Design review of the part built by this model. Coordinates are the model's own, in mm. A direction names the side the tool comes from. Round coordinates to 2 decimals unless told otherwise and drop trailing zeros. Loops run counter-clockwise (first coordinate to the right, second up) from the corner with the lowest first, then second, coordinate; pieces in that order, holes last. Notation, with made-up numbers: (37, 14.25) -> (91, 14.25) arc R7 ccw to (91, 20.25) -> close; hole circle Ø2 at (-39.75, 18). An arc over 180 degrees is marked (long way). Use a Markdown table: item, result. Add a question column.
from build123d import *

# Parameters (mm, degrees)
SALIENTE_EXTRUIR1_DEPTH = 4
CORTAR_EXTRUIR4_DEPTH   = 5
CROQUIS10_R             = 1.5
CORTAR_EXTRUIR5_DEPTH   = 5
CROQUIS12_R             = 2.575
CORTAR_EXTRUIR6_DEPTH   = 5


with BuildPart() as part:
    # Croquis1 → Saliente-Extruir1 (new body)
    with BuildSketch(Plane(origin=(0, 0, 0), x_dir=(1, 0, 0), z_dir=(0, 1, 0))):
        with BuildLine():
            Line((-18.025, -25), (18.025, -25))
            ThreePointArc((18.025, -25), (21.560533906, -23.535533906), (23.025, -20))
            Line((23.025, -20), (23.025, -14))
            Line((23.025, -14), (29.025, -14))
            Line((29.025, -14), (29.025, -8))
            Line((29.025, -8), (23.025, -8))
            Line((23.025, -8), (23.025, -1.55))
            Line((23.025, -1.55), (20.975, -1.55))
            Line((20.975, -1.55), (20.975, -2.8))
            Line((20.975, -2.8), (18.075, -2.8))
            Line((18.075, -2.8), (18.075, -1.55))
            Line((18.075, -1.55), (16.025, -1.55))
            Line((16.025, -1.55), (16.025, 1.55))
            Line((16.025, 1.55), (18.075, 1.55))
            Line((18.075, 1.55), (18.075, 2.8))
            Line((18.075, 2.8), (20.975, 2.8))
            Line((20.975, 2.8), (20.975, 1.55))
            Line((20.975, 1.55), (23.025, 1.55))
            Line((23.025, 1.55), (23.025, 8))
            Line((23.025, 8), (29.025, 8))
            Line((29.025, 8), (29.025, 14))
            Line((29.025, 14), (23.025, 14))
            Line((23.025, 14), (23.025, 20))
            ThreePointArc((23.025, 20), (21.560533906, 23.535533906), (18.025, 25))
            Line((18.025, 25), (-18.025, 25))
            ThreePointArc((-18.025, 25), (-21.560533906, 23.535533906), (-23.025, 20))
            Line((-23.025, 20), (-23.025, -20))
            ThreePointArc((-23.025, -20), (-21.560533906, -23.535533906), (-18.025, -25))
        make_face()
    extrude(amount=SALIENTE_EXTRUIR1_DEPTH)

    # Croquis7 → Cortar-Extruir4 (cut, through all)
    with BuildSketch(Plane(origin=(0, 4, 0), x_dir=(1, 0, 0), z_dir=(0, 1, 0))):
        with BuildLine():
            Line((21.402341989, 1.55), (23.025, 1.55))
            Line((23.025, 1.55), (23.025, -1.55))
            Line((23.025, -1.55), (21.402341989, -1.55))
            ThreePointArc((21.402341989, -1.55), (20.900478098, -2.869619136), (19.525, -3.187930349))
            ThreePointArc((19.525, -3.187930349), (18.280747615, -2.971867524), (17.642475162, -1.882163243))
            ThreePointArc((17.642475162, -1.882163243), (16.05076038, -1.575149398), (15.66772275, 0))
            ThreePointArc((15.66772275, 0), (16.05076038, 1.575149398), (17.642475162, 1.882163243))
            ThreePointArc((17.642475162, 1.882163243), (18.280747615, 2.971867524), (19.525, 3.187930349))
            ThreePointArc((19.525, 3.187930349), (20.900478098, 2.869619136), (21.402341989, 1.55))
        make_face()
    extrude(amount=-CORTAR_EXTRUIR4_DEPTH, mode=Mode.SUBTRACT)

    # Croquis10 → Cortar-Extruir5 (cut, through all)
    with BuildSketch(Plane(origin=(0, 4, 0), x_dir=(1, 0, 0), z_dir=(0, 1, 0))):
        with Locations((24.085660172, 15.060660172)):
            Circle(CROQUIS10_R)
        with Locations((24.085660172, 6.939339828)):
            Circle(CROQUIS10_R)
        with Locations((24.085660172, -15.060660172)):
            Circle(CROQUIS10_R)
        with Locations((24.085660172, -6.939339828)):
            Circle(CROQUIS10_R)
    extrude(amount=-CORTAR_EXTRUIR5_DEPTH, mode=Mode.SUBTRACT)

    # Croquis12 → Cortar-Extruir6 (cut, through all)
    with BuildSketch(Plane(origin=(0, 4, 0), x_dir=(1, 0, 0), z_dir=(0, 1, 0))):
        with Locations((-17.525, 16)):
            Circle(CROQUIS12_R)
        with Locations((-8.525, 16)):
            Circle(CROQUIS12_R)
        with Locations((-8.525, 9)):
            Circle(CROQUIS12_R)
        with Locations((-17.525, 9)):
            Circle(CROQUIS12_R)
    extrude(amount=-CORTAR_EXTRUIR6_DEPTH, mode=Mode.SUBTRACT)


solid = part.part
1. Consider section D-D on y = 0.75. Give the number of separate pieces and of enclosed holes in the cut face, plus the area to 3 significant figures.
2. Consider section C-C on x = 24. State the section outline as (y, z) points.
3. Consider section B-B on z = -15. State the section outline as (x, y) points (3 decimals).
4. Mouldability with a two-part tool opening along Z and no side actions: class faces 1 (the face through (23.025, 2, 4)), 2 (the face through (21.599, 1.972, -23.496)), 3 (the face through (23.025, 2, 18)) as +Z half, -Z half, draft (parallel to the pull), parting line (faces both ways), or undercut.
5. For faces 4 (the face through (29.025, 2, 11)), 5 (the face through (27, 2, 8)), list the 3-axis set-ups (+Z, -Z, +X, -X, +Y, -Y) from which the entire face can be reached by the end or side of a thin tool; tool diameter is ignored.
6. Insertion check: P1, Ø1.3, axis at x = 22, y = 2, coming from the +Z side; P2, Ø2, axis at y = 2, z = -5, coming from the +X side (3 decimals); P3, Ø1.8, axis at x = 22, y = 2, coming from the -Z side. Each pin has a flat end and moves straight along its axis. Give the tip position at first contact, or say it passes through.
7. To check wall thickness, follow probe 1 along X at (y, z) = (2.3, -9) (3 decimals); probe 2 along Z at (x, y) = (-19, 2.1); probe 3 along X at (y, z) = (1.85, -16) (3 decimals). State the ranges of each line that lie inside material, in increasing order. Write a range as from..to.
8. Consider section A-A on x = -16.5. State the section outline as (y, z) points, plus the area to 3 significant figures.
Verdict:
| question | item | result |
|---|---|---|
| 1 | separate pieces | 1 |
| 1 | enclosed holes | 4 |
| 1 | area | 2,230 mm² |
| 2 | outline | (0, -13.56) -> (4, -13.56) -> (4, -8.44) -> (0, -8.44) -> close; (0, 8.44) -> (4, 8.44) -> (4, 13.56) -> (0, 13.56) -> close |
| 3 | outline | (-23.025, 0) -> (-19.898, 0) -> (-19.898, 4) -> (-23.025, 4) -> close; (-15.152, 0) -> (-10.898, 0) -> (-10.898, 4) -> (-15.152, 4) -> close; (-6.152, 0) -> (22.587, 0) -> (22.587, 4) -> (-6.152, 4) -> close |
| 4 | face 1 | undercut |
| 4 | face 2 | -Z half |
| 4 | face 3 | draft |
| 5 | face 4 | +Z, -Z, +X, +Y, -Y |
| 5 | face 5 | +X, +Y, -Y |
| 6 | P1 | stops at z = 23.73 |
| 6 | P2 | stops at x = 23.025 |
| 6 | P3 | stops at z = -23.94 |
| 7 | probe 1 | x = -23.025..-20.1, -14.95..-11.1, -5.95..29.025 |
| 7 | probe 2 | z = -24.9..-18.11, -13.89..-11.11, -6.89..24.9 |
| 7 | probe 3 | x = -23.025..-20.1, -14.95..-11.1, -5.95..22.916 |
| 8 | outline | (0, -25) -> (4, -25) -> (4, -18.36) -> (0, -18.36) -> close; (0, -13.64) -> (4, -13.64) -> (4, -11.36) -> (0, -11.36) -> close; (0, -6.64) -> (4, -6.64) -> (4, 25) -> (0, 25) -> close |
| 8 | area | 162 mm² |
